```python
from build123d import *

# Parameters (mm, degrees)
SKETCH_1_W          = 29
SKETCH_1_H          = 19.2
EXTRUDE_1_DEPTH     = 7.5
SKETCH_2_R          = 1.6
CUT_EXTRUDE_1_DEPTH = 19.938320939
SKETCH_3_W          = 25
SKETCH_3_H          = 3
CUT_EXTRUDE_2_DEPTH = 7.5
SKETCH_4_R          = 1.6
CUT_EXTRUDE_3_DEPTH = 26.201984049
SKETCH_6_W          = 29
SKETCH_6_H          = 6.5
CUT_EXTRUDE_5_DEPTH = 19.938320939
SKETCH_7_R          = 2.6
SKETCH_7_R_2        = 1.6
CUT_EXTRUDE_6_DEPTH = 1.5


with BuildPart() as part:
    # 草图1 → 凸台-拉伸1 (new body)
    with BuildSketch(Plane.XY):
        Rectangle(SKETCH_1_W, SKETCH_1_H)
    extrude(amount=EXTRUDE_1_DEPTH)

    # 草图2 → 切除-拉伸1 (cut, through all)
    with BuildSketch(Plane.XY.offset(7.5)):
        with Locations((10, -6.1)):
            Circle(SKETCH_2_R)
        with Locations((-10, -6.1)):
            Circle(SKETCH_2_R)
    extrude(amount=-CUT_EXTRUDE_1_DEPTH, mode=Mode.SUBTRACT)

    # 草图3 → 切除-拉伸2 (cut)
    with BuildSketch(Plane.XY.offset(7.5)):
        with Locations((0, -1.0394817)):
            Rectangle(SKETCH_3_W, SKETCH_3_H)
    extrude(amount=-CUT_EXTRUDE_2_DEPTH, mode=Mode.SUBTRACT)

    # 草图4 → 切除-拉伸3 (cut, through all)
    with BuildSketch(Plane.XZ.offset(9.6)):
        with Locations(Location((-5.5, 3.75, 0), (0, 0, 270))):
            Circle(SKETCH_4_R)
        with Locations(Location((5.5, 3.75, 0), (0, 0, 270))):
            Circle(SKETCH_4_R)
    extrude(amount=-CUT_EXTRUDE_3_DEPTH, mode=Mode.SUBTRACT)

    # 草图6 → 切除-拉伸5 (cut, through all)
    with BuildSketch(Plane.XY.offset(7.5)):
        with Locations((0, 6.35)):
            Rectangle(SKETCH_6_W, SKETCH_6_H)
    extrude(amount=-CUT_EXTRUDE_5_DEPTH, mode=Mode.SUBTRACT)

    # 草图7 → 切除-拉伸6 (cut)
    # profile 1 of 2: a face of its own
    with BuildSketch(Plane.XZ.offset(9.6)):
        with Locations(Location((-5.5, 3.75, 0), (0, 0, 270))):
            Circle(SKETCH_7_R)
        with Locations(Location((-5.5, 3.75, 0), (0, 0, 270))):
            Circle(SKETCH_7_R_2, mode=Mode.SUBTRACT)
    # profile 2 of 2: a face of its own
    with BuildSketch(Plane.XZ.offset(9.6)):
        with Locations(Location((5.5, 3.75, 0), (0, 0, 270))):
            Circle(SKETCH_7_R)
        with Locations(Location((5.5, 3.75, 0), (0, 0, 270))):
            Circle(SKETCH_7_R_2, mode=Mode.SUBTRACT)
    extrude(amount=-CUT_EXTRUDE_6_DEPTH, mode=Mode.SUBTRACT)


solid = part.part
```
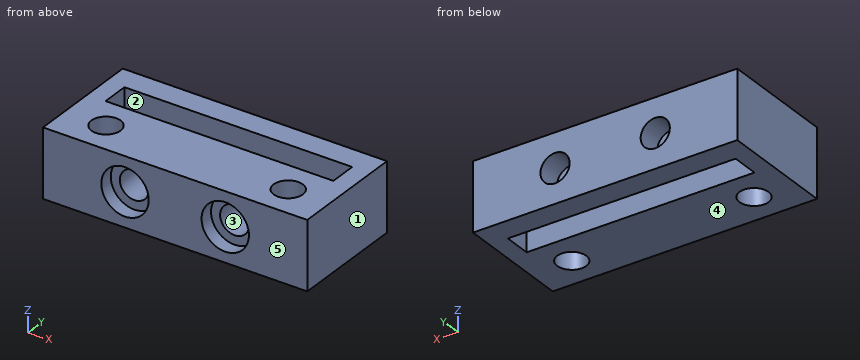
Read the model definition and answer for the solid it produces. Units are mm, in the model's axes. Face numbers are marked on the shaded views. A direction names the side the tool comes from. Give positions to 0.01 mm unless a question says otherwise; leave off trailing zeros. Order: outer loops, then holes, each group sorted by start corner. A loop starts at its lowest first (then second) coordinate and runs counter-clockwise, first axis right, second up.
(1) Find section A-A (x = -5.5). Give the vertices of the cut face in (y, z).
(2) Given pin 1 (3.5 mm diameter, centred on x = 5.5, z = 3.75, fed in from -Y); pin 2 (2.5 mm diameter, centred on x = 10, y = -6.1, fed in from +Z), each flat-ended and moving along its own axis, determine where each tip first touches the part or whether it passes through.
(3) Straight lines are drawn through the part: L1, parallel to X at y = 1.9, z = 3.75; L2, parallel to Y at x = -10, z = 3; L3, parallel to Y at x = 4, z = 0.5. For each, find the intervals that lie inside material, in ascending order.
(4) Find section D-D (x = -1.75). Give the vertices of the cut face in (y, z), plus the area to 4 significant figures.
(5) For the marked faces 1 and 2, determine the directions among +Z, -Z, +X, -X, +Y, -Y from which every point of the face is accessible in a straight line to the end or side of a thin tool.
(6) For a pull along Z with two mould halves and no side action, classify the marked faces 3, 4 and 5 as released by +Z, released by -Z, zero draft, split by the parting line, or undercut.
(7) Find section C-C (y = -5.5). Give the vertices of the cut face in (x, z), plus the area to 3 significant figures.
(8) Find section B-B (z = 3.75). Give the number of separate pieces and of enclosed holes in the cut face, plus the area to 3 significant figures.
Result sheet:
1. outline: (-9.6, 0) - (-2.54, 0) - (-2.54, 2.15) - (-8.1, 2.15) - (-8.1, 1.15) - (-9.6, 1.15) - close; (-9.6, 6.35) - (-8.1, 6.35) - (-8.1, 5.35) - (-2.54, 5.35) - (-2.54, 7.5) - (-9.6, 7.5) - close; (0.46, 0) - (3.1, 0) - (3.1, 2.15) - (0.46, 2.15) - close; (0.46, 5.35) - (3.1, 5.35) - (3.1, 7.5) - (0.46, 7.5) - close
2. pin 1: stops at y = -8.1
2. pin 2: passes through
3. L1: x = -14.5 to -7.1, -3.9 to 3.9, 7.1 to 14.5
3. L2: y = -9.6 to -7.7, -4.5 to -2.54, 0.46 to 3.1
3. L3: y = -9.6 to -2.54, 0.46 to 3.1
4. outline: (-9.6, 0) - (-2.54, 0) - (-2.54, 7.5) - (-9.6, 7.5) - close; (0.46, 0) - (3.1, 0) - (3.1, 7.5) - (0.46, 7.5) - close
4. area: 72.75 mm2
5. face 1: +Z, -Z, +X, +Y, -Y
5. face 2: +Z, -Z
6. face 3: undercut
6. face 4: released by -Z
6. face 5: zero draft
7. outline: (-14.5, 0) - (-11.48, 0) - (-11.48, 7.5) - (-14.5, 7.5) - close; (-8.52, 0) - (8.52, 0) - (8.52, 7.5) - (-8.52, 7.5) - close; (11.48, 0) - (14.5, 0) - (14.5, 7.5) - (11.48, 7.5) - close; hole circle Ø3.2 at (-5.5, 3.75); hole circle Ø3.2 at (5.5, 3.75)
7. area: 157 mm2
8. separate pieces: 4
8. enclosed holes: 2
8. area: 209 mm2
